Here's how the part is built. I have some questions about the finished solid (model axes, mm). Face numbers are marked on the shaded views. Give positions to 0.01 mm unless a question says otherwise; leave off trailing zeros. Write each loop counter-clockwise with the first axis right and the second up, starting at its lowest first coordinate (ties: lowest second). Pieces come first, ordered by that corner, then holes. Notation, with made-up numbers: (85, 77) -> (131, 77) arc R4 ccw to (131, 84) -> close; hole circle Ø5 at (-10, 35). An arc over 180 degrees is marked (long way). Return JSON: item names as keys, results as strings.
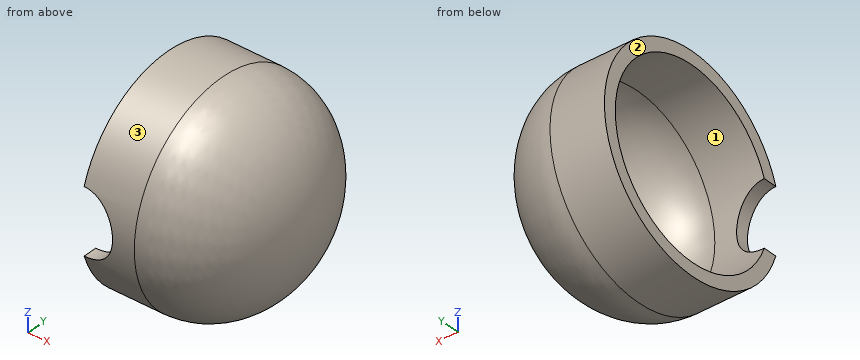
from build123d import *

# Parameters (mm, degrees)
SKETCH1_R               = 4.85
BOSS_EXTRUDE1_DEPTH     = 2.5
DOME1_FACE_RADIUS       = 4.85
DOME1_HEIGHT            = 4
SHELL1_T                = -0.6
CUT_EXTRUDE2_DEPTH      = 4
CUT_EXTRUDE2_DEPTH_BACK = 4
SKETCH4_R               = 1.5


with BuildPart() as part:
    # Sketch1 → Boss-Extrude1 (new body)
    with BuildSketch(Plane(origin=(0, 0, 0), x_dir=(0, 0, -1), z_dir=(1, 0, 0))):
        with Locations((-8.491927182, 4.785070814)):
            Circle(SKETCH1_R)
    extrude(amount=BOSS_EXTRUDE1_DEPTH)

    # Dome1: an elliptical dome of height H over a round flat face of radius A is half a spheroid: the quarter ellipse of half axes A and H revolved about the face's axis
    with BuildSketch(Plane((2.5, 4.785070814, 8.491927182), x_dir=(0, 0, 1), z_dir=(0, 1, 0)), mode=Mode.PRIVATE) as dome1_quarter:
        Ellipse(DOME1_FACE_RADIUS, DOME1_HEIGHT)
        Rectangle(DOME1_FACE_RADIUS, DOME1_HEIGHT, align=(Align.MIN, Align.MIN), mode=Mode.INTERSECT)
    revolve(dome1_quarter.sketch, axis=Axis((2.5, 4.785070814, 8.491927182), (1, 0, 0)))

    # Shell1
    shell1_openings = [part.faces().sort_by_distance(p)[0] for p in [
        (0, 4.785070814, 8.491927182),
    ]]
    offset(amount=SHELL1_T, openings=shell1_openings, kind=Kind.INTERSECTION)

    # Sketch4 → Cut-Extrude2 (cut, two sides: drawn at the far end of the back side and taken through both)
    with BuildSketch(Plane(origin=(0, 0, 0), x_dir=(1, 0, 0), z_dir=(0, 1, 0)).offset(-CUT_EXTRUDE2_DEPTH_BACK)):
        with Locations((0, -8.491927182)):
            Circle(SKETCH4_R)
    extrude(amount=CUT_EXTRUDE2_DEPTH + CUT_EXTRUDE2_DEPTH_BACK, mode=Mode.SUBTRACT)


solid = part.part
1. For pin 1 Ø4 at (y, z) = (2, 8.5) entering from +X; pin 2 Ø1 at (y, z) = (8, 10) entering from +X; pin 3 Ø1.5 at (x, y) = (4, 6.5) entering from +Z, each with a flat end and sliding along its axis, tell me the tip position at first contact or that it passes through.
Taken from the geometry:
{"pin 1": "stops at x = 6.45", "pin 2": "stops at x = 5.61", "pin 3": "stops at z = 13.05"}
2. If we mould it in two halves opening along Z, with no side actions, what happens to the marked faces 1, 2 and 3? For each: released by +Z, released by -Z, zero draft, split by the parting line, or undercut.
Taken from the geometry:
{"face 1": "undercut", "face 2": "zero draft", "face 3": "split by the parting line"}
3. Suppose I cut it at A-A, the plane x = 2. List the corners of the cut face in (y, z) for me.
Taken from the geometry:
{"outline": "circle Ø9.7 at (4.79, 8.49); hole circle Ø8.5 at (4.79, 8.49)"}
4. If I drill on line 1 (Y direction, x = 2, z = 8); line 2 (Z direction, x = 1.25, y = 1.5); line 3 (Z direction, x = 1, y = 2.5), over which ranges is the centre line in solid material (lowest first)? Write a range as [from, to].
Taken from the geometry:
{"line 1": "y = [-0.04, 0.56], [9.01, 9.61]", "line 2": "z = [4.92, 5.8], [11.19, 12.06]", "line 3": "z = [4.21, 4.91], [12.08, 12.77]"}
